Autodesk Inventor part; units mm, degrees
ref_plane "Start plane" through (0, 0, 20) normal (0, 0, 1) x (1, 0, 0)
ref_plane "End plane" through (0, 0, 480) normal (0, 0, 1) x (1, 0, 0)
ref_plane "Work Plane4" through (700, -16.1, 480) normal (0, 0, 1) x (1, 0, 0)
ref_plane "Start plane" through (0, 0, 20) normal (0, 0, 1) x (1, 0, 0)
ref_plane "End plane" through (0, 0, 480) normal (0, 0, 1) x (1, 0, 0)
sketch "Sketch" plane through (0, 0, 0) normal (0, 0, 1) x (1, 0, 0)
  line L0 (-20, -16.1) -> (-20, 16.1)
  line L1 (-16.1, 20) -> (16.1, 20)
  line L2 (20, 16.1) -> (20, -16.1)
  line L3 (16.1, -20) -> (-16.1, -20)
  arc A0 (-20, -16.1) -> (-16.1, -20) centre (-16.1, -16.1) ccw
  arc A1 (-16.1, 20) -> (-20, 16.1) centre (-16.1, 16.1) ccw
  arc A2 (20, 16.1) -> (16.1, 20) centre (16.1, 16.1) ccw
  arc A3 (16.1, -20) -> (20, -16.1) centre (16.1, -16.1) ccw
  line L4 (-14.8, 17.4) -> (14.8, 17.4)
  line L5 (17.4, 14.8) -> (17.4, -14.8)
  line L6 (14.8, -17.4) -> (-14.8, -17.4)
  line L7 (-17.4, -14.8) -> (-17.4, 14.8)
  line L8 (0, 29.1308) -> (0, -29.1308) construction
  line L9 (-29.1308, 0) -> (29.1308, 0) construction
  arc A4 (-17.4, -14.8) -> (-14.8, -17.4) centre (-14.8, -14.8) ccw
  arc A5 (-14.8, 17.4) -> (-17.4, 14.8) centre (-14.8, 14.8) ccw
  arc A6 (17.4, 14.8) -> (14.8, 17.4) centre (14.8, 14.8) ccw
  arc A7 (14.8, -17.4) -> (17.4, -14.8) centre (14.8, -14.8) ccw
  dimension "d7" = 3.9
  dimension "d10" = 40
  dimension "d11" = 40
  dimension "d12" = 2.6
  dimension "d15" = 20
  dimension "d16" = 20
  dimension "d19" = 2.6
  dimension "d20" = 2.6
extrude "Body" add sketch "Sketch" along normal up to surface (460 mm away) from surface at 20
sketch "Sketch3" plane through (0, 0, 0) normal (0, 0, 1) x (1, 0, 0)
  line L0 (0, 0) -> (10, 0)
ref_plane "Work Plane3" through (0, 0, 0) normal (0, -1, 0) x (1, 0, 0)
sketch "Sketch4" plane through (0, 0, 0) normal (0, -1, 0) x (1, 0, 0)
  line L0 (-2, 20) -> (12, 20)
  line L1 (-2, 480) -> (12, 480)
  dimension "d18" = 460
ref_plane "Work Plane4" through (700, -16.1, 480) normal (0, 0, 1) x (1, 0, 0)
split "Split1" plane through (700, -16.1, 480) removes the side toward (0, 0, 1)
ref_plane "Work Plane5" through (-800, -16.1, 20) normal (0, 0, -1) x (-1, 0, 0)
split "Split2" plane through (-800, -16.1, 20) removes the side toward (0, 0, -1)
equation "\"d7\" = G_IR"
equation "\"d10\" = G_H"
equation "\"d11\" = G_W"
equation "\"d12\" = G_T"
equation "\"d15\" = 0.5 * d10"
equation "\"d16\" = 0.5 * d11"
equation "\"d19\" = G_T"
equation "\"d20\" = G_T"
equation "\"d3\" = G_L"
equation "\"G_W\" = 40"
equation "\"G_H\" = 40"
equation "\"G_T\" = 2.6"
equation "\"G_IR\" = 3.9"
equation "\"G_L\" = d18"
properties part number "EN 10210-2 - 40 x 40 x 2.6 - 460" material "Steel, Galvanized"
The listing builds one solid part. Answer for the finished solid, in the listing's coordinates (mm). A direction names the side the tool comes from. Coordinates: 2 decimals unless noted, no trailing zeros. Write each loop counter-clockwise with the first axis right and the second up, starting at its lowest first coordinate (ties: lowest second). Pieces come first, ordered by that corner, then holes. Notation, with made-up numbers: (22, 2.5) -> (43, 2.5) arc R15 cw to (43, 21.5) -> close; hole circle Ø11 at (39.5, 28). An arc over 180 degrees is marked (long way). Write each question's results on one line, items separated by ' | '. Start each with the question number.
1) A tool of negligible diameter and unlimited length cuts with its end or side. For faces 4 (the flat face through (-18, 0, 20)), 5 (the flat face through (0, -17.4, 247)), from which of +Z, -Z, +X, -X, +Y, -Y can it reach the whole face along a straight path? Write none if from no direction.
2) A cutting plane is placed at B-B (z = 441.5). Determine the outline of the cut face in (x, y), then the cut area to 3 significant figures.
3) Straight lines are drawn through the part: probe 1 along X at (y, z) = (-5, 70); probe 2 along Y at (x, z) = (16, 400). For each, find the intervals that lie inside material, in ascending order.
4) For a pull along Y with two mould halves and no side action, classify faces 1 (the flat face through (0, 17.4, 247)), 2 (the flat face through (0, 20, 247)), 3 (the flat face through (-20, 0, 247)) as +Y half, -Y half, draft (parallel to the pull), parting line (faces both ways), or undercut.
5) A cutting plane is placed at A-A (x = -7.5). Determine the outline of the cut face in (y, z), then the cut area to 3 significant figures.
6) Flat-ended cylindrical pins translate along their axes: pin 1 Ø8 at (x, y) = (-13.5, -3) entering from +Z; pin 2 Ø3 at (x, y) = (10, -14.5) entering from -Z. Find the tip coordinate at first contact, or state that the pin passes through.
Values follow:
1) face 4: -Z, +X, -X, +Y, -Y | face 5: +Z, -Z
2) outline: (-20, -16.1) arc R3.9 ccw to (-16.1, -20) -> (16.1, -20) arc R3.9 ccw to (20, -16.1) -> (20, 16.1) arc R3.9 ccw to (16.1, 20) -> (-16.1, 20) arc R3.9 ccw to (-20, 16.1) -> close; hole (-17.4, -14.8) arc R2.6 ccw to (-14.8, -17.4) -> (14.8, -17.4) arc R2.6 ccw to (17.4, -14.8) -> (17.4, 14.8) arc R2.6 ccw to (14.8, 17.4) -> (-14.8, 17.4) arc R2.6 ccw to (-17.4, 14.8) -> close | area: 382 mm²
3) probe 1: -20 to -17.4, 17.4 to 20 | probe 2: -20 to -17.11, 17.11 to 20
4) face 1: undercut | face 2: +Y half | face 3: draft
5) outline: (-20, 20) -> (-17.4, 20) -> (-17.4, 480) -> (-20, 480) -> close; (17.4, 20) -> (20, 20) -> (20, 480) -> (17.4, 480) -> close | area: 2,390 mm²
6) pin 1: z = 480 | pin 2: through
